Geometry check sheet. Reference: the model listing, model coordinates, mm. A direction names the side the tool comes from. Give positions to 0.01 mm unless a question says otherwise; leave off trailing zeros. Loops run counter-clockwise (first coordinate to the right, second up) from the corner with the lowest first, then second, coordinate; pieces in that order, holes last. Notation, with made-up numbers: (15, -3) -> (74, -3) arc R5 ccw to (74, 3) -> close; hole circle Ø10 at (-22, 80). An arc over 180 degrees is marked (long way). Write each question's results on one line, items separated by ' | '. Start each with the question number.
1) Scan lines: line 1 (Y direction, x = -133, z = 356) (3 decimals); line 2 (Y direction, x = -133.35, z = 357.4) (1 decimal); line 3 (Y direction, x = 35.5, z = 162.5). Record each from-to range of solid material in increasing order. Write a range as from..to.
2) Depth check by flat-ended pin: pin 1 (4 mm diameter, centred on x = 107.5, y = 299, fed in from +Z); pin 2 (14.5 mm diameter, centred on x = -139.5, y = 306, fed in from +Z); pin 3 (1.5 mm diameter, centred on x = -35.5, z = 199, fed in from +Y). Enter the tip coordinate at first touch or a pass-through.
3) Draft check along Y on faces 6 (the face through (2, 165.1, 378)), 7 (the face through (1, 469.9, 17)), 8 (the face through (-134, 299, 355.6)). Enter one of: pulls with the +Y half, pulls with the -Y half, needs draft (parallel to the pull), parting line crosses it, or undercut.
4) Sectioned sample at C-C on x = 157.5. Record the cut outline in (y, z) (3 decimals), then the cut area to 3 significant figures.
5) Sectioned sample at D-D on z = 208.5. Record the cut outline in (x, y), then the cut area to 3 significant figures.
6) Sectioned sample at A-A on z = 116.5. Record the cut outline in (x, y), then the cut area to 3 significant figures.
7) Sectioned sample at B-B on y = 238. Record the cut outline in (x, z).
8) Set-up check for faces 1 (the face through (2.49, 337.17, 5.43)), 2 (the face through (-127, 387, 59)), 3 (the face through (127, 178, 378)), 4 (the face through (128, 301, 358.14)), 5 (the face through (-127, 330, 126)): record each of +Z, -Z, +X, -X, +Y, -Y from which the full face is reachable in a straight line by a thin tool's end or side.
```python
from build123d import *

# Parameters (mm, degrees)
SKETCH1_W           = 393.7
SKETCH1_H           = 342.9
BOSS_EXTRUDE1_DEPTH = 355.6
SKETCH2_W           = 50.8
SKETCH2_H           = 44.45
BOSS_EXTRUDE2_DEPTH = 2.54
BOSS_EXTRUDE3_DEPTH = 2.54
SKETCH4_R           = 3.81
CUT_EXTRUDE1_DEPTH  = 2.54
BOSS_EXTRUDE4_DEPTH = 50.8
FILLET1_R           = 6.35
FILLET2_R           = 6.35
SKETCH6_R           = 14.2875
SKETCH6_R_2         = 11.1125
CUT_EXTRUDE2_DEPTH  = 2.54
FILLET3_R           = 19.05
BOSS_EXTRUDE5_DEPTH = 127
FILLET4_R           = 39.116
SKETCH8_W           = 254
SKETCH8_H           = 63.5
CUT_EXTRUDE3_DEPTH  = 25.4


with BuildPart() as part:
    # Sketch1 → Boss-Extrude1 (new body)
    with BuildSketch(Plane.XY):
        with Locations((0, 171.45)):
            Rectangle(SKETCH1_W, SKETCH1_H)
    extrude(amount=BOSS_EXTRUDE1_DEPTH)

    # Sketch2 → Boss-Extrude2 (add)
    with BuildSketch(Plane.XY.offset(355.6)):
        with Locations((-133.35, 298.45)):
            Rectangle(SKETCH2_W, SKETCH2_H)
    extrude(amount=BOSS_EXTRUDE2_DEPTH)

    # Sketch3 → Boss-Extrude3 (add)
    with BuildSketch(Plane.XY.offset(355.6)):
        with BuildLine():
            Line((88.9, 307.975), (165.1, 307.975))
            ThreePointArc((165.1, 307.975), (174.625, 298.45), (165.1, 288.925))
            Line((165.1, 288.925), (88.9, 288.925))
            ThreePointArc((88.9, 288.925), (79.375, 298.45), (88.9, 307.975))
        make_face()
    extrude(amount=BOSS_EXTRUDE3_DEPTH)

    # Sketch4 → Cut-Extrude1 (cut)
    with BuildSketch(Plane.XY.offset(358.14)):
        with Locations((92.075, 298.45)):
            Circle(SKETCH4_R)
        with Locations((108.286467636, 298.45)):
            Circle(SKETCH4_R)
        with Locations((124.497935272, 298.45)):
            Circle(SKETCH4_R)
    extrude(amount=-CUT_EXTRUDE1_DEPTH, mode=Mode.SUBTRACT)

    # Sketch5 → Boss-Extrude4 (add)
    with BuildSketch(Plane.XY.offset(355.6)):
        with BuildLine():
            Line((-114.3, 190.5), (114.3, 190.5))
            ThreePointArc((114.3, 190.5), (127, 177.8), (114.3, 165.1))
            Line((114.3, 165.1), (-114.3, 165.1))
            ThreePointArc((-114.3, 165.1), (-127, 177.8), (-114.3, 190.5))
        make_face()
    extrude(amount=BOSS_EXTRUDE4_DEPTH)

    # Fillet1
    fillet1_edges = [part.edges().sort_by_distance(p)[0] for p in [
        (-127, 177.8, 406.4),
        (0, 165.1, 406.4),
        (127, 177.8, 406.4),
        (0, 190.5, 406.4),
    ]]
    fillet(fillet1_edges, radius=FILLET1_R)

    # Fillet2
    fillet2_edges = [part.edges().sort_by_distance(p)[0] for p in [
        (-107.95, 276.225, 356.87),
        (-107.95, 320.675, 356.87),
        (-158.75, 320.675, 356.87),
        (-158.75, 276.225, 356.87),
    ]]
    fillet(fillet2_edges, radius=FILLET2_R)

    # Sketch6 → Cut-Extrude2 (cut)
    # profile 1 of 2: a face of its own
    with BuildSketch(Plane.XY.offset(358.14)):
        with Locations((-133.35, 296.545)):
            Circle(SKETCH6_R)
        with Locations((-133.35, 296.545)):
            Circle(SKETCH6_R_2, mode=Mode.SUBTRACT)
    # profile 2 of 2: a face of its own
    with BuildSketch(Plane.XY.offset(358.14)):
        with BuildLine():
            Line((-134.9375, 296.545), (-134.9375, 315.595))
            ThreePointArc((-134.9375, 315.595), (-133.35, 317.1825), (-131.7625, 315.595))
            Line((-131.7625, 315.595), (-131.7625, 296.545))
            ThreePointArc((-131.7625, 296.545), (-133.35, 294.9575), (-134.9375, 296.545))
        make_face()
    extrude(amount=-CUT_EXTRUDE2_DEPTH, mode=Mode.SUBTRACT)

    # Fillet3
    fillet3_edges = [part.edges().sort_by_distance(p)[0] for p in [
        (196.85, 171.45, 355.6),
        (0, 342.9, 355.6),
        (-196.85, 171.45, 355.6),
        (0, 342.9, 0),
        (196.85, 171.45, 0),
        (0, 0, 0),
        (-196.85, 171.45, 0),
        (0, 0, 355.6),
        (-196.85, 342.9, 177.8),
        (196.85, 342.9, 177.8),
        (196.85, 0, 177.8),
        (-196.85, 0, 177.8),
    ]]
    fillet(fillet3_edges, radius=FILLET3_R)

    # Sketch7 → Boss-Extrude5 (add, symmetric)
    with BuildSketch(Plane(origin=(0, 0, 0), x_dir=(0, 0, -1), z_dir=(1, 0, 0))):
        Polygon((-65.877338054, 342.9), (-3.487013452, 469.9), (-31.786520589, 469.9), (-94.17684519, 342.9), align=None)
    extrude(amount=BOSS_EXTRUDE5_DEPTH, both=True)

    # Fillet4
    fillet4_edges = [part.edges().sort_by_distance(p)[0] for p in [
        (-127, 469.9, 17.636767021),
        (127, 469.9, 17.636767021),
    ]]
    fillet(fillet4_edges, radius=FILLET4_R)

    # Sketch8 → Cut-Extrude3 (cut)
    with BuildSketch(Plane(origin=(0, 342.9, 0), x_dir=(1, 0, 0), z_dir=(0, 1, 0))):
        with Locations((0, -125.92684519)):
            Rectangle(SKETCH8_W, SKETCH8_H)
    extrude(amount=-CUT_EXTRUDE3_DEPTH, mode=Mode.SUBTRACT)


solid = part.part
```
Result:
1) line 1: 276.225..282.262, 285.438..294.997, 317.143..320.675 | line 2: 276.2..282.3, 285.4..295, 317.2..320.7 | line 3: 0..342.9
2) pin 1: z = 355.6 | pin 2: z = 358.14 | pin 3: y = 342.9
3) face 6: pulls with the -Y half | face 7: pulls with the +Y half | face 8: undercut
4) outline: (0, 19.05) arc R19.05 ccw to (19.05, 0) -> (323.85, 0) arc R19.05 ccw to (342.9, 19.05) -> (342.9, 336.55) arc R19.05 ccw to (323.85, 355.6) -> (307.975, 355.6) -> (307.975, 358.14) -> (288.925, 358.14) -> (288.925, 355.6) -> (19.05, 355.6) arc R19.05 ccw to (0, 336.55) -> close | area: 122,000 mm^2
5) outline: (-196.85, 19.05) arc R19.05 ccw to (-177.8, 0) -> (177.8, 0) arc R19.05 ccw to (196.85, 19.05) -> (196.85, 323.85) arc R19.05 ccw to (177.8, 342.9) -> (-177.8, 342.9) arc R19.05 ccw to (-196.85, 323.85) -> close | area: 135,000 mm^2
6) outline: (-196.85, 19.05) arc R19.05 ccw to (-177.8, 0) -> (177.8, 0) arc R19.05 ccw to (196.85, 19.05) -> (196.85, 323.85) arc R19.05 ccw to (177.8, 342.9) -> (127, 342.9) -> (127, 317.5) -> (-127, 317.5) -> (-127, 342.9) -> (-177.8, 342.9) arc R19.05 ccw to (-196.85, 323.85) -> close | area: 128,000 mm^2
7) outline: (-196.85, 19.05) arc R19.05 ccw to (-177.8, 0) -> (177.8, 0) arc R19.05 ccw to (196.85, 19.05) -> (196.85, 336.55) arc R19.05 ccw to (177.8, 355.6) -> (-177.8, 355.6) arc R19.05 ccw to (-196.85, 336.55) -> close
8) face 1: -Z, +X, -X | face 2: +Z, -Z, -X, +Y | face 3: +Z, +X | face 4: +Z, +X, -X, +Y | face 5: +Y
